```python
from build123d import *

# Parameters (mm, degrees)
SCHIZZO1_W                   = 60
SCHIZZO1_H                   = 60
ESTRUSIONE_ESTRUSIONE1_DEPTH = 60.2
SCHIZZO2_R                   = 7.6
TAGLIO_ESTRUSIONE1_DEPTH     = 105.038646666
SCHIZZO3_R                   = 7.6
TAGLIO_ESTRUSIONE2_DEPTH     = 105.038646666
SCHIZZO4_W                   = 18
SCHIZZO4_H                   = 60
TAGLIO_ESTRUSIONE3_DEPTH     = 35


with BuildPart() as part:
    # Schizzo1 → Estrusione-Estrusione1 (new body)
    with BuildSketch(Plane.XY):
        with Locations((-30, 30)):
            Rectangle(SCHIZZO1_W, SCHIZZO1_H)
    extrude(amount=ESTRUSIONE_ESTRUSIONE1_DEPTH)

    # Schizzo2 → Taglio-Estrusione1 (cut, through all)
    with BuildSketch(Plane(origin=(0, 0, 0), x_dir=(0, 0, -1), z_dir=(1, 0, 0))):
        with Locations((-13.6, 30)):
            Circle(SCHIZZO2_R)
    extrude(amount=-TAGLIO_ESTRUSIONE1_DEPTH, mode=Mode.SUBTRACT)

    # Schizzo3 → Taglio-Estrusione2 (cut, through all)
    with BuildSketch(Plane(origin=(0, 60, 0), x_dir=(0, 0, -1), z_dir=(0, 1, 0))):
        with Locations(Location((-47.2, 30, 0), (0, 0, 180))):
            Circle(SCHIZZO3_R)
    extrude(amount=-TAGLIO_ESTRUSIONE2_DEPTH, mode=Mode.SUBTRACT)

    # Schizzo4 → Taglio-Estrusione3 (cut)
    with BuildSketch(Plane.XY.offset(60.2)):
        with Locations((-51, 30)):
            Rectangle(SCHIZZO4_W, SCHIZZO4_H)
        with Locations((-9, 30)):
            Rectangle(SCHIZZO4_W, SCHIZZO4_H)
    extrude(amount=-TAGLIO_ESTRUSIONE3_DEPTH, mode=Mode.SUBTRACT)


solid = part.part
```
Part model, mm, in its own coordinate system. A direction names the side the tool comes from. Round coordinates to 2 decimals unless told otherwise and drop trailing zeros. Write each loop counter-clockwise with the first axis right and the second up, starting at its lowest first coordinate (ties: lowest second). Pieces come first, ordered by that corner, then holes.
Item 1: Cut at C-C, the plane y = 45.5. Give the cut face in (x, z).
Results:
outline: (-60, 0) - (0, 0) - (0, 25.2) - (-18, 25.2) - (-18, 60.2) - (-42, 60.2) - (-42, 25.2) - (-60, 25.2) - close; hole circle Ø15.2 at (-30, 47.2)
Item 2: Which spindle directions (+Z, -Z, +X, -X, +Y, -Y) get a long thin tool onto all of the face, cutting with end or side? Do faces 5 (the flat face through (-30, 30, 0)), 6 (the flat face through (-18, 30, 43)). Say none if no direction does.
Results:
face 5: -Z, +X, -X, +Y, -Y
face 6: +Z, +X, +Y, -Y
Item 3: Cut at A-A, the plane x = -30. Give the cut face in (y, z), plus the area to 3 significant figures.
Results:
outline: (0, 0) - (60, 0) - (60, 39.6) - (0, 39.6) - close; (0, 54.8) - (60, 54.8) - (60, 60.2) - (0, 60.2) - close; hole circle Ø15.2 at (30, 13.6)
area: 2,520 mm2
Item 4: Two-plate mould, pull along X, no slides. Class faces 1 (the flat face through (-42, 30, 43)), 2 (the flat face through (0, 23, 10)), 3 (the cylindrical face through (-24.86, 30.42, 41.6)), 4 (the flat face through (-51, 30, 25.2)): +X half, -X half, draft (parallel to the pull), parting line (faces both ways), or undercut.
Results:
face 1: -X half
face 2: +X half
face 3: undercut
face 4: draft
Item 5: Drop flat-ended pins along their axis: pin 1 Ø10 at (y, z) = (36, 37.5) entering from -X; pin 2 Ø2 at (x, y) = (-12, 39) entering from +Z. Give the stop position or say it passes through.
Results:
pin 1: stops at x = -42
pin 2: stops at z = 25.2
Item 6: Cut at D-D, the plane y = 34. Give the cut face in (x, z).
Results:
outline: (-60, 0) - (0, 0) - (0, 7.14) - (-60, 7.14) - close; (-60, 20.06) - (0, 20.06) - (0, 25.2) - (-18, 25.2) - (-18, 60.2) - (-42, 60.2) - (-42, 25.2) - (-60, 25.2) - close; hole circle Ø15.2 at (-30, 47.2)
Item 7: Cut at B-B, the plane z = 47.2. Give the cut face in (x, y), plus the area to 3 significant figures.
Results:
outline: (-42, 0) - (-37.6, 0) - (-37.6, 60) - (-42, 60) - close; (-22.4, 0) - (-18, 0) - (-18, 60) - (-22.4, 60) - close
area: 528 mm2
Item 8: Probe L1, parallel to Y at x = -37.5, z = 13.6; L2, parallel to X at y = 12, z = 47; L3, parallel to Z at x = -46.5, y = 19. List the from-to ranges inside material, lowest first.
Results:
L1: y = 0 to 22.4, 37.6 to 60
L2: x = -42 to -37.6, -22.4 to -18
L3: z = 0 to 25.2
